from build123d import *

# Parameters (mm, degrees)
BOX360_W          = 72
BOX360_H          = 35
BOX360_DEPTH      = 3
BOX361_W          = 3
BOX361_H          = 35
BOX361_DEPTH      = 72
CYLINDER019_R     = 35
CYLINDER019_DEPTH = 36
CYLINDER010_R     = 58
CYLINDER010_DEPTH = 36
FILLET003_R       = 10.5
FILLET012_R       = 6


with BuildPart() as cube360:
    # Box360 → Box360 (new body)
    with BuildSketch(Plane(origin=(-36, 1, -1.5), x_dir=(1, 0, 0), z_dir=(0, 0, 1))):
        with Locations((36, 17.5)):
            Rectangle(BOX360_W, BOX360_H)
    extrude(amount=BOX360_DEPTH)


with BuildPart() as fusion019:
    # Box361 → Box361 (new body)
    with BuildSketch(Plane(origin=(-1.5, 1, -36), x_dir=(1, 0, 0), z_dir=(0, 0, 1))):
        with Locations((1.5, 17.5)):
            Rectangle(BOX361_W, BOX361_H)
    extrude(amount=BOX361_DEPTH)

    # Fusion019: union Cube360
    add(cube360.part)


with BuildPart() as cylinder019:
    # Cylinder019 → Cylinder019 (new body)
    with BuildSketch(Plane(origin=(0, 0, 0), x_dir=(1, 0, 0), z_dir=(0, 1, 0))):
        Circle(CYLINDER019_R)
    extrude(amount=CYLINDER019_DEPTH)


with BuildPart() as front_wheel_inner_120mm:
    # Cylinder010 → Cylinder010 (new body)
    with BuildSketch(Plane(origin=(0, 0, 0), x_dir=(1, 0, 0), z_dir=(0, 1, 0))):
        Circle(CYLINDER010_R)
    extrude(amount=CYLINDER010_DEPTH)

    # Fillet003
    fillet003_edges = [front_wheel_inner_120mm.edges().sort_by_distance(p)[0] for p in [
        (-58, 0, 0),
        (-58, 36, 0),
    ]]
    fillet(fillet003_edges, radius=FILLET003_R)

    # Cut004026018020024: cut Cylinder019
    add(cylinder019.part, mode=Mode.SUBTRACT)

    # Fillet012
    fillet012_edges = [front_wheel_inner_120mm.edges().sort_by_distance(p)[0] for p in [
        (-35, 36, 0),
        (-35, 0, 0),
    ]]
    fillet(fillet012_edges, radius=FILLET012_R)

    # Cut004026018020025: cut Fusion019
    add(fusion019.part, mode=Mode.SUBTRACT)


with BuildPart() as front_wheel_inner_120mm_1:
    # Cut004026018020025 placement: moved
    add(front_wheel_inner_120mm.part.moved(Location((185, 0, 0))))


solid = front_wheel_inner_120mm_1.part
Check sheet for the modelled part. Datum: model origin and axes. Units: mm. A direction names the side the tool comes from. Round coordinates to 2 decimals unless told otherwise and drop trailing zeros. Loops run counter-clockwise (first coordinate to the right, second up) from the corner with the lowest first, then second, coordinate; pieces in that order, holes last. Notation, with made-up numbers: (-20.5, 15.25) -> (-8.5, 15.25) arc R18 cw to (-8.5, 35.25) -> close; hole circle Ø3 at (51, 44). An arc over 180 degrees is marked (long way). Put each result on its own line as item: value. Start each with the question number.
1. Section check C-C (x = 185). Enter the section's corners in (y, z).
2. Section check B-B (y = 13). Enter the section's corners in (x, z), plus the area to 3 significant figures.
3. Scan lines: probe 1 along Z at (x, y) = (211.5, 18); probe 2 along X at (y, z) = (13, -18); probe 3 along X at (y, z) = (25, -22). Record each from-to range of solid material in increasing order.
4. Gauge pin test, flat ends, axial feed: pin 1 (6 mm diameter, centred on x = 155, y = 26, fed in from -Z); pin 2 (2.5 mm diameter, centred on x = 184.5, y = 17, fed in from +Z); pin 3 (2.5 mm diameter, centred on x = 184.5, y = 16, fed in from -Z); pin 4 (3.5 mm diameter, centred on y = 20.5, z = 0.5, fed in from -X). Record the tip position at first contact, or that the pin passes through.
5. Access from +Z, -Z, +X, -X, +Y, -Y to the whole of each face (thin tool, end or side, straight path). Record for faces 4 (the face through (146, 36, 14)), 5 (the face through (185, 18, -36)).
6. Section check A-A (z = 0). Enter the section's corners in (x, y), plus the area to 3 significant figures.
7. Draft check along Z on faces 1 (the face through (146, 0, 14)), 2 (the face through (209.49, 17.832, 25.005)), 3 (the face through (138.97, 17.9, 35.29)). Enter one of: +Z half, -Z half, draft (parallel to the pull), parting line (faces both ways), or undercut.
Findings:
1. outline: (0, -47.5) arc R10.5 ccw to (10.5, -58) -> (25.5, -58) arc R10.5 ccw to (36, -47.5) -> (36, -41) arc R6 ccw to (33.32, -36) -> (2.68, -36) arc R6 ccw to (0, -41) -> close; (0, 41) arc R6 ccw to (2.68, 36) -> (33.32, 36) arc R6 ccw to (36, 41) -> (36, 47.5) arc R10.5 ccw to (25.5, 58) -> (10.5, 58) arc R10.5 ccw to (0, 47.5) -> close
2. outline: circle Ø116 at (185, 0); hole (149, -1.5) -> (150.03, -1.5) arc R35 ccw to (183.5, -34.97) -> (183.5, -36) -> (186.5, -36) -> (186.5, -34.97) arc R35 ccw to (219.97, -1.5) -> (221, -1.5) -> (221, 1.5) -> (219.97, 1.5) arc R35 ccw to (186.5, 34.97) -> (186.5, 36) -> (183.5, 36) -> (183.5, 34.97) arc R35 ccw to (150.03, 1.5) -> (149, 1.5) -> close
2. area: 6,710 mm^2
3. probe 1: z = -51.59 to -22.86, 22.86 to 51.59
3. probe 2: x = 129.86 to 154.98, 215.02 to 240.14
3. probe 3: x = 131.33 to 157.78, 212.22 to 238.67
4. pin 1: stops at z = -51.32
4. pin 2: stops at z = 58
4. pin 3: stops at z = -58
4. pin 4: stops at x = 127
5. face 4: +Z, -Z, +X, -X, +Y
5. face 5: +Y, -Y
6. outline: (127, 10.5) arc R10.5 ccw to (137.5, 0) -> (144, 0) arc R6 ccw to (149, 2.68) -> (149, 33.32) arc R6 ccw to (144, 36) -> (137.5, 36) arc R10.5 ccw to (127, 25.5) -> close; (221, 2.68) arc R6 ccw to (226, 0) -> (232.5, 0) arc R10.5 ccw to (243, 10.5) -> (243, 25.5) arc R10.5 ccw to (232.5, 36) -> (226, 36) arc R6 ccw to (221, 33.32) -> close
6. area: 1,470 mm^2
7. face 1: draft
7. face 2: undercut
7. face 3: parting line
